Could you check a few things on this model? Use its own coordinates, in mm. Face numbers are marked on the shaded views. A direction names the side the tool comes from. Coordinates: 2 decimals unless noted, no trailing zeros. Order: outer loops, then holes, each group sorted by start corner. A loop starts at its lowest first (then second) coordinate and runs counter-clockwise, first axis right, second up. Notation, with made-up numbers: (-11.75, -22.5) - (35.25, -22.5) arc R34 ccw to (35.25, 9.5) - close; hole circle Ø10 at (-30, 16). An arc over 180 degrees is marked (long way). Answer as a JSON object with one key per item and string values. Group by question number.
(1) Please list where these lines run through material, in increasing order: probe 1 along X at (y, z) = (2.05, 0); probe 2 along X at (y, z) = (3.25, 4); probe 3 along Y at (x, z) = (17, -1.5).
(2) Will these pins go through, and if not, where does the flat tip stop? P1, Ø0.6, axis at y = 5.5, z = 3.5, coming from the +X side; P2, Ø1.9, axis at y = 6, z = 3.5, coming from the -X side; P3, Ø4, axis at x = 1, z = -3, coming from the -Y side; P4, Ø1.5, axis at x = 33, y = 1, coming from the -Z side.
(3) Imagine slicing it at B-B, the plane z = 0. Write out the boundary of the cut face in (x, y), and give its area (4 significant figures).
(4) Imagine slicing it at A-A, the plane y = 6.5. Write out the boundary of the cut face in (x, z), and give its area (3 significant figures).
(5) Imagine slicing it at C-C, the plane x = 13.5. Write out the boundary of the cut face in (y, z).
(6) Which directions (+Z, -Z, +X, -X, +Y, -Y) give clear straight access to the entire face, cutting with the end or side of a thin tool? Please do the marked faces 1, 2, 3, 4 and 5.
(7) We'd pull the mould along Z, two halves only. Please class the marked faces 6, 7 and 8: pulls with the +Z half, pulls with the -Z half, needs draft (parallel to the pull), parting line crosses it, or undercut.
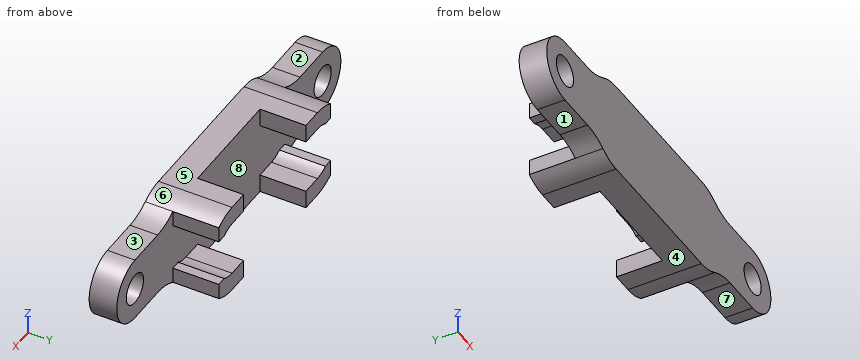
from build123d import *

# Parameters (mm, degrees)
SKETCH2_R           = 1.65
BOSS_EXTRUDE1_DEPTH = 3
BOSS_EXTRUDE2_DEPTH = 5


with BuildPart() as part:
    # Sketch2 → Boss-Extrude1 (new body)
    with BuildSketch(Plane(origin=(0, 0, 0), x_dir=(1, 0, 0), z_dir=(0, 1, 0))):
        with BuildLine():
            Line((0, 3.5), (4.356739527, 3.5))
            ThreePointArc((4.356739527, 3.5), (5.879286162, 3.704522124), (7.293887604, 4.303588328))
            ThreePointArc((7.293887604, 4.303588328), (8.519819988, 4.822755522), (9.839300635, 5))
            Line((9.839300635, 5), (26.260699365, 5))
            ThreePointArc((26.260699365, 5), (27.580180012, 4.822755522), (28.806112396, 4.303588328))
            ThreePointArc((28.806112396, 4.303588328), (30.220713838, 3.704522124), (31.743260473, 3.5))
            Line((31.743260473, 3.5), (36.1, 3.5))
            ThreePointArc((36.1, 3.5), (39.6, 0), (36.1, -3.5))
            Line((36.1, -3.5), (31.743260473, -3.5))
            ThreePointArc((31.743260473, -3.5), (30.220713838, -3.704522124), (28.806112396, -4.303588328))
            ThreePointArc((28.806112396, -4.303588328), (27.580180012, -4.822755522), (26.260699365, -5))
            Line((26.260699365, -5), (9.839300635, -5))
            ThreePointArc((9.839300635, -5), (8.519819988, -4.822755522), (7.293887604, -4.303588328))
            ThreePointArc((7.293887604, -4.303588328), (5.879286162, -3.704522124), (4.356739527, -3.5))
            Line((4.356739527, -3.5), (0, -3.5))
            ThreePointArc((0, -3.5), (-3.5, 0), (0, 3.5))
        make_face()
        with Locations(Location((0, 0, 0), (0, 0, 270))):
            Circle(SKETCH2_R, mode=Mode.SUBTRACT)
        with Locations(Location((36.1, 0, 0), (0, 0, 270))):
            Circle(SKETCH2_R, mode=Mode.SUBTRACT)
    extrude(amount=BOSS_EXTRUDE1_DEPTH)

    # Sketch3 → Boss-Extrude2 (add)
    with BuildSketch(Plane(origin=(0, 3, 0), x_dir=(1, 0, 0), z_dir=(0, 1, 0))):
        with BuildLine():
            Line((7.293887604, 4.303588328), (7.293887604, 2.582152997))
            Line((7.293887604, 2.582152997), (8.312052816, 2.582152997))
            ThreePointArc((8.312052816, 2.582152997), (9.047612247, 2.893653313), (9.839300635, 3))
            Line((9.839300635, 3), (12.05, 3))
            Line((12.05, 3), (12.05, 5))
            Line((12.05, 5), (9.839300635, 5))
            ThreePointArc((9.839300635, 5), (8.519819988, 4.822755522), (7.293887604, 4.303588328))
        make_face()
        with BuildLine():
            Line((28.806112396, 4.303588328), (28.806112396, 2.582152997))
            Line((28.806112396, 2.582152997), (27.787947184, 2.582152997))
            ThreePointArc((27.787947184, 2.582152997), (27.052387753, 2.893653313), (26.260699365, 3))
            Line((26.260699365, 3), (24.05, 3))
            Line((24.05, 3), (24.05, 5))
            Line((24.05, 5), (26.260699365, 5))
            ThreePointArc((26.260699365, 5), (27.580180012, 4.822755522), (28.806112396, 4.303588328))
        make_face()
        with BuildLine():
            Line((9.839300635, -3), (12.05, -3))
            Line((12.05, -3), (12.05, -5))
            Line((12.05, -5), (9.839300635, -5))
            ThreePointArc((9.839300635, -5), (8.519819988, -4.822755522), (7.293887604, -4.303588328))
            Line((7.293887604, -4.303588328), (7.293887604, -2.582152997))
            Line((7.293887604, -2.582152997), (8.312052816, -2.582152997))
            ThreePointArc((8.312052816, -2.582152997), (9.047612247, -2.893653313), (9.839300635, -3))
        make_face()
        with BuildLine():
            Line((27.787947184, -2.582152997), (28.806112396, -2.582152997))
            Line((28.806112396, -2.582152997), (28.806112396, -4.303588328))
            ThreePointArc((28.806112396, -4.303588328), (27.580180012, -4.822755522), (26.260699365, -5))
            Line((26.260699365, -5), (24.05, -5))
            Line((24.05, -5), (24.05, -3))
            Line((24.05, -3), (26.260699365, -3))
            ThreePointArc((26.260699365, -3), (27.052387753, -2.893653313), (27.787947184, -2.582152997))
        make_face()
    extrude(amount=BOSS_EXTRUDE2_DEPTH)


solid = part.part
Result set:
{
 "1": {"probe 1": "x = -3.5 to -1.65, 1.65 to 34.45, 37.75 to 39.6", "probe 2": "x = 7.29 to 12.05, 24.05 to 28.81", "probe 3": "y = 0 to 3"},
 "2": {"P1": "stops at x = 28.81", "P2": "stops at x = 7.29", "P3": "stops at y = 0", "P4": "stops at z = -3.5"},
 "3": {"outline": "(-3.5, 0) - (-1.65, 0) - (-1.65, 3) - (-3.5, 3) - close; (1.65, 0) - (34.45, 0) - (34.45, 3) - (1.65, 3) - close; (37.75, 0) - (39.6, 0) - (39.6, 3) - (37.75, 3) - close", "area": "109.5 mm^2"},
 "4": {"outline": "(7.29, -4.3) arc R5 ccw to (9.84, -5) - (12.05, -5) - (12.05, -3) - (9.84, -3) arc R3 cw to (8.31, -2.58) - (7.29, -2.58) - close; (7.29, 2.58) - (8.31, 2.58) arc R3 cw to (9.84, 3) - (12.05, 3) - (12.05, 5) - (9.84, 5) arc R5 ccw to (7.29, 4.3) - close; (24.05, -5) - (26.26, -5) arc R5 ccw to (28.81, -4.3) - (28.81, -2.58) - (27.79, -2.58) arc R3 cw to (26.26, -3) - (24.05, -3) - close; (24.05, 3) - (26.26, 3) arc R3 cw to (27.79, 2.58) - (28.81, 2.58) - (28.81, 4.3) arc R5 ccw to (26.26, 5) - (24.05, 5) - close", "area": "38.3 mm^2"},
 "5": {"outline": "(0, -5) - (3, -5) - (3, 5) - (0, 5) - close"},
 "6": {"face 1": "-Z, -X, +Y, -Y", "face 2": "+Z, -X, +Y, -Y", "face 3": "+Z, +X, +Y, -Y", "face 4": "-Z, +X, -X, +Y, -Y", "face 5": "+Z, +X, -X, +Y, -Y"},
 "7": {"face 6": "pulls with the +Z half", "face 7": "pulls with the -Z half", "face 8": "undercut"}
}
